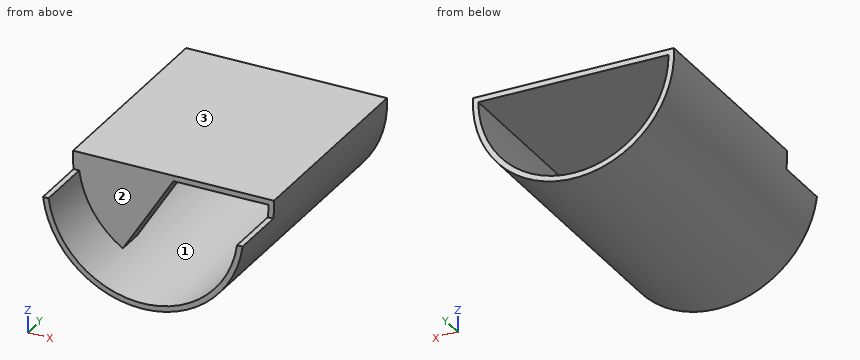
```python
from build123d import *

# Parameters (mm, degrees)
BOSS_EXTRUDE1_DEPTH = 150
SKETCH3_W           = 109.836241742
SKETCH3_H           = 14
CUT_EXTRUDE3_DEPTH  = 5
CUT_EXTRUDE4_DEPTH  = 10
BOSS_EXTRUDE2_DEPTH = 15
DRAFT2_ANGLE        = 60


with BuildPart() as part:
    # Sketch1 → Boss-Extrude1 (new body)
    with BuildSketch(Plane(origin=(0, 0, 0), x_dir=(1, 0, 0), z_dir=(0, 1, 0))):
        with BuildLine():
            Line((-54.918120871, -3), (54.918120871, -3))
            ThreePointArc((54.918120871, -3), (0, 55), (-54.918120871, -3))
        make_face()
        with BuildLine():
            Line((-52, 0), (52, 0))
            ThreePointArc((52, 0), (0, 52), (-52, 0))
        make_face(mode=Mode.SUBTRACT)
    extrude(amount=BOSS_EXTRUDE1_DEPTH)

    # Sketch3 → Cut-Extrude3 (cut)
    with BuildSketch(Plane.XY.offset(3)):
        with Locations((0, 25)):
            Rectangle(SKETCH3_W, SKETCH3_H)
    extrude(amount=-CUT_EXTRUDE3_DEPTH, mode=Mode.SUBTRACT)

    # Sketch4 → Cut-Extrude4 (cut)
    with BuildSketch(Plane.XY.offset(3)):
        Polygon((0, 0), (62.110162625, 0), (62.110162625, 32), (-64.723211538, 32), (-64.723211538, 0), align=None)
    extrude(amount=-CUT_EXTRUDE4_DEPTH, mode=Mode.SUBTRACT)

    # Sketch6 → Boss-Extrude2 (add)
    with BuildSketch(Plane(origin=(0, 32, 0), x_dir=(-1, 0, 0), z_dir=(0, -1, 0))):
        with BuildLine():
            Line((27.712812921, 44), (0, 0))
            Line((0, 0), (52, 0))
            ThreePointArc((52, 0), (45.525082492, 25.129004438), (27.712812921, 44))
        make_face()
    extrude(amount=-BOSS_EXTRUDE2_DEPTH)

    # Draft2
    draft2_faces = [part.faces().sort_by_distance(p)[0] for p in [
        (-29.079569776, 47, -16.051385257),
    ]]
    draft(draft2_faces, Plane(origin=(-27.712812921, 47, -44), x_dir=(0.5329387100211931, 0, 0.8461538461538461), z_dir=(0.8461538461538461, 0, -0.5329387100211931)), DRAFT2_ANGLE)


solid = part.part
```
Source: CAD feature listing. Evaluate the final solid. Frame: model axes, mm. Face numbers are marked on the shaded views. Give positions to 0.01 mm unless a question says otherwise; leave off trailing zeros. Loops run counter-clockwise (first coordinate to the right, second up) from the corner with the lowest first, then second, coordinate; pieces in that order, holes last. Notation, with made-up numbers: (6, -17.5) -> (34, -17.5) arc R38 ccw to (34, 21.5) -> close; hole circle Ø1 at (-16, 69). An arc over 180 degrees is marked (long way). Use a Markdown table: item, result. Add a question column.
(1) Section query A-A (z = -28). Output: boundary loops of the cut face in (x, y), then the cut area to 3 significant figures.
(2) Section query C-C (y = 73). Output: boundary loops of the cut face in (x, z), then the cut area to 3 significant figures.
(3) First-contact query: pin 1 Ø2.5 at (x, y) = (-53, 12.5) entering from +Z; pin 2 Ø23.5 at (x, z) = (-19.5, -22.5) entering from -Y; pin 3 Ø1 at (x, y) = (12.5, 23) entering from +Z. Flat tips, straight axial feed; report the tip coordinate or a pass-through.
(4) Pull-direction query (Z, two-part tool) for the marked faces 1, 2 and 3; classes: +Z half, -Z half, draft (parallel to the pull), parting line (faces both ways), or undercut.
(5) Section query B-B (x = 41.5). Output: boundary loops of the cut face in (y, z), then the cut area to 3 significant figures.
(6) Ray query, line 1 (X direction, y = 93, z = -21); line 2 (Z direction, x = -41, y = 78); line 3 (Z direction, x = 42.5, y = 92). Return the intervals inside material, ascending.
(7) Section query D-D (z = -42). Output: boundary loops of the cut face in (x, y), then the cut area to 3 significant figures.
Checked values:
| question | item | result |
|---|---|---|
| 1 | outline | (-47.34, 0) -> (-43.82, 0) -> (-43.82, 32) -> (-17.64, 32) -> (-17.64, 47) -> (-43.82, 85.37) -> (-43.82, 150) -> (-47.34, 150) -> close; (43.82, 0) -> (47.34, 0) -> (47.34, 150) -> (43.82, 150) -> close |
| 1 | area | 1,950 mm^2 |
| 2 | outline | (-54.92, 3) arc R55 ccw (long way) to (54.92, 3) -> close; hole (-39.23, -34.13) arc R52 ccw to (52, 0) -> (-17.74, 0) -> close |
| 2 | area | 1,500 mm^2 |
| 3 | pin 1 | z = -7 |
| 3 | pin 2 | y = 32 |
| 3 | pin 3 | z = -50.35 |
| 4 | face 1 | undercut |
| 4 | face 2 | draft |
| 4 | face 3 | +Z half |
| 5 | outline | (0, -36.09) -> (150, -36.09) -> (150, -31.33) -> (0, -31.33) -> close; (32, 0) -> (150, 0) -> (150, 3) -> (32, 3) -> close |
| 5 | area | 1,070 mm^2 |
| 6 | line 1 | -50.83 to -44.61, 47.57 to 50.83 |
| 6 | line 2 | -36.66 to -31.98, -31.51 to 3 |
| 6 | line 3 | -34.91 to -29.96, 0 to 3 |
| 7 | outline | (-35.51, 0) -> (-30.66, 0) -> (-30.66, 32) -> (-26.45, 32) -> (-26.45, 47) -> (-30.66, 53.16) -> (-30.66, 150) -> (-35.51, 150) -> close; (30.66, 0) -> (35.51, 0) -> (35.51, 150) -> (30.66, 150) -> close |
| 7 | area | 1,530 mm^2 |
